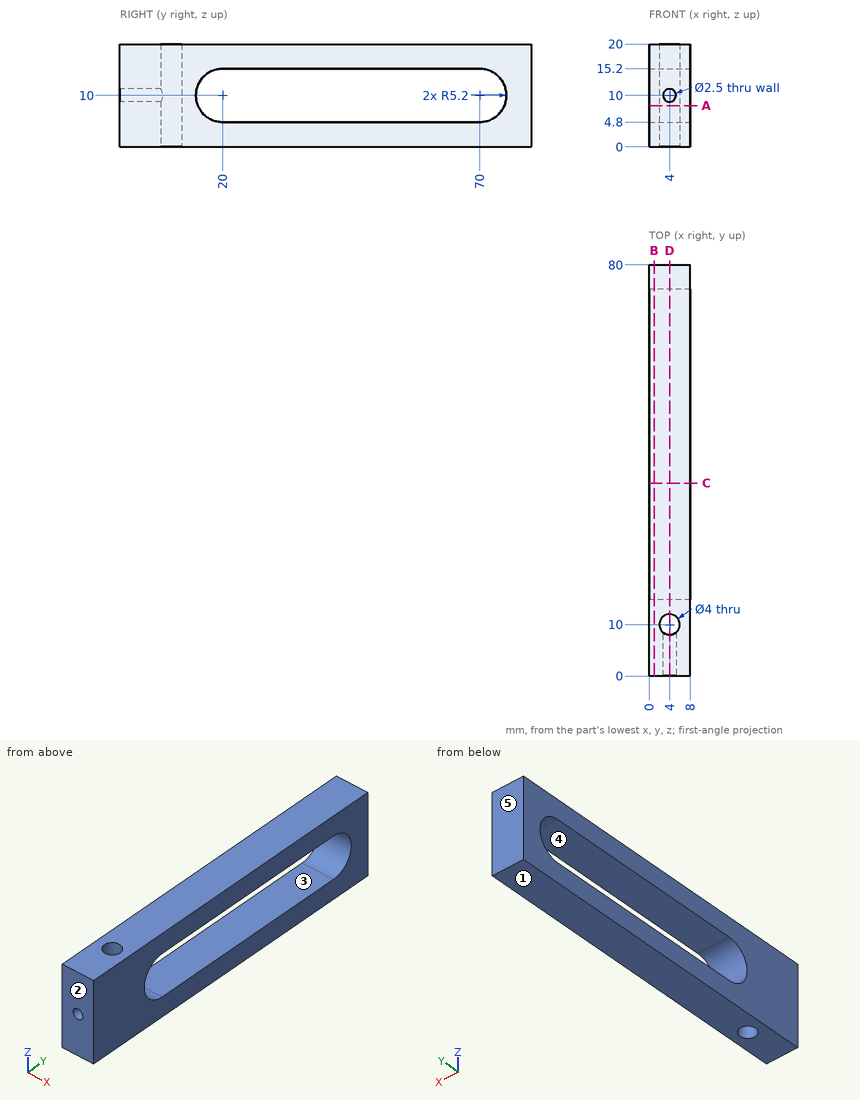
Job drawing, mm, ordinate dimensions from the low corner. One solid piece. A direction names the side the tool comes from. Round coordinates to 2 decimals unless told otherwise and drop trailing zeros. Loops run counter-clockwise (first coordinate to the right, second up) from the corner with the lowest first, then second, coordinate; pieces in that order, holes last.
(1) Which spindle directions (+Z, -Z, +X, -X, +Y, -Y) get a long thin tool onto all of the face, cutting with end or side? Do the marked faces 4 and 5. Say none if no direction does.
(2) Cut at A-A (z = 8). Give the cut face in (x, y).
(3) Two-plate mould, pull along Z, no slides. Class the marked faces 1, 2 and 3: +Z half, -Z half, draft (parallel to the pull), parting line (faces both ways), or undercut.
(4) Wall check: line 1 along Z through (x, y) = (6.5, 23); line 2 along Y through (x, z) = (5.75, 10); line 3 along Y through (x, z) = (4, 14.75). Give the ranges that are in metal, low to high.
(5) Drop a flat-ended pin along its axis: pin 1 (2.5 mm diameter, centred on x = 4, y = 10, fed in from +Z). Give the stop position or say it passes through.
(6) Cut at B-B (x = 1). Give the cut face in (y, z), plus the area to 3 significant figures.
(7) Cut at C-C (y = 37.5). Give the cut face in (x, z).
(8) Cut at D-D (x = 4). Give the cut face in (y, z), plus the area to 3 significant figures.
Findings below:
1. face 4: +X, -X
1. face 5: +Z, -Z, +X, -X, +Y
2. outline: (0, 0) - (8, 0) - (8, 15.2) - (0, 15.2) - close; (0, 74.8) - (8, 74.8) - (8, 80) - (0, 80) - close; hole circle Ø4 at (4, 10)
3. face 1: -Z half
3. face 2: draft
3. face 3: undercut
4. line 1: z = 0 to 4.8, 15.2 to 20
4. line 2: y = 0 to 9.03, 10.97 to 14.8, 75.2 to 80
4. line 3: y = 0 to 8, 12 to 17.88, 72.12 to 80
5. pin 1: passes through
6. outline: (0, 0) - (80, 0) - (80, 20) - (0, 20) - close; hole (20, 4.8) - (70, 4.8) arc R5.2 ccw to (70, 15.2) - (20, 15.2) arc R5.2 ccw to start
6. area: 995 mm2
7. outline: (0, 0) - (8, 0) - (8, 4.8) - (0, 4.8) - close; (0, 15.2) - (8, 15.2) - (8, 20) - (0, 20) - close
8. outline: (0, 0) - (8, 0) - (8, 8.75) - (0, 8.75) - close; (0, 11.25) - (8, 11.25) - (8, 20) - (0, 20) - close; (12, 0) - (80, 0) - (80, 20) - (12, 20) - close; hole (20, 4.8) - (70, 4.8) arc R5.2 ccw to (70, 15.2) - (20, 15.2) arc R5.2 ccw to start
8. area: 895 mm2
